Design review of the part built by this model. Coordinates are the model's own, in mm. Face numbers are marked on the shaded views. A direction names the side the tool comes from. Round coordinates to 2 decimals unless told otherwise and drop trailing zeros. Loops run counter-clockwise (first coordinate to the right, second up) from the corner with the lowest first, then second, coordinate; pieces in that order, holes last. Notation, with made-up numbers: M 38,-17 L 96,-17 A8 cw 96,-12 Z; hole C 10,75 d3. An arc over 180 degrees is marked long. Answer as CSV lines item,"result". Start each with the question number.
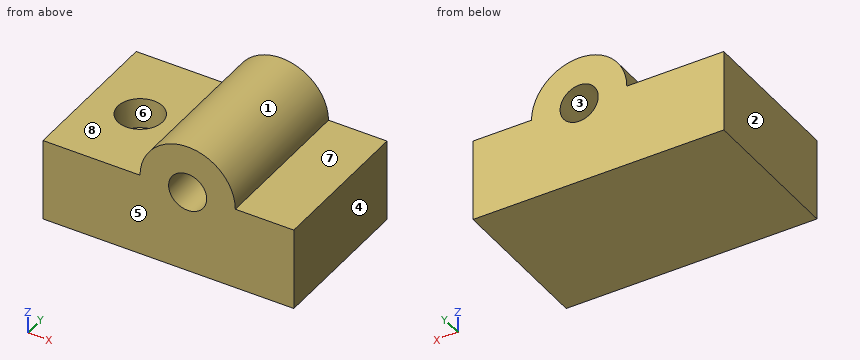
from build123d import *

# Parameters (mm, degrees)
F1_DEPTH = 60
F2_R     = 7.5
F3_DEPTH = 60
F5_R     = 8.827636
F6_DEPTH = 12


with BuildPart() as f1:
    # F0 (on Front) → F1 (new body)
    with BuildSketch(Plane.XZ):
        with BuildLine():
            Line((-98.720774, 0), (0, 0))
            Line((0, 0), (0, 32.434803))
            Line((0, 32.434803), (-22.520235, 32.434803))
            Line((-22.520235, 32.434803), (-23.024651, 32.434803))
            ThreePointArc((-23.024651, 32.434803), (-41.782826, 51.192978), (-60.541002, 32.434803))
            Line((-60.541002, 32.434803), (-61.611962, 32.434803))
            Line((-61.611962, 32.434803), (-98.720774, 32.434803))
            Line((-98.720774, 32.434803), (-98.720774, 0))
        make_face()
    extrude(amount=F1_DEPTH)

    # F2 (on face) → F3 (cut, through all)
    with BuildSketch(Plane.XZ.offset(60)):
        with Locations((-41.782826, 32.434803)):
            Circle(F2_R)
    extrude(amount=-F3_DEPTH, mode=Mode.SUBTRACT)

    # F5 (on face) → F6 (cut)
    with BuildSketch(Plane.XY.offset(32.434803)):
        with Locations((-78.823261, -29.944986)):
            Circle(F5_R)
    extrude(amount=-F6_DEPTH, mode=Mode.SUBTRACT)


solid = f1.part
Item 1: Consider section B-B, the plane y = -20. Write out the cut boundary in (x, z), then the cut area to 3 significant figures.
Item 2: Consider section D-D, the plane z = 47. Write out the cut boundary in (x, y), then the cut area to 3 significant figures.
Item 3: To check wall thickness, follow line 1 (X direction, y = -25.5, z = 28.5); line 2 (X direction, y = -17, z = 33); line 3 (Z direction, x = -8, y = -11.5). State the ranges of each line that lie inside material, in increasing order.
Item 4: Tool access review of the marked faces 4, 5, 6, 7 and 8: name each direction out of +Z, -Z, +X, -X, +Y, -Y from which nothing blocks a thin tool from reaching the whole face with its end or side.
Item 5: Consider section C-C, the plane x = -12. Write out the cut boundary in (y, z), then the cut area to 3 significant figures.
Item 6: Consider section A-A, the plane z = 29. Write out the cut boundary in (x, y), then the cut area to 3 significant figures.
Item 7: The part is to be moulded in two halves that separate along X. For the marked faces 1, 2 and 3, say which applies: +X half, -X half, draft (parallel to the pull), parting line (faces both ways), or undercut.
Item 8: Insertion check: pin 1 Ø4 at (y, z) = (-9, 41.5) entering from -X; pin 2 Ø20.5 at (x, y) = (-78.82, -29.94) entering from +Z. Each pin has a flat end and moves straight along its axis. Give the tip position at first contact, or say it passes through.
Found:
1,outline,"M -98.72,0 L 0,0 L 0,32.43 L -23.02,32.43 A18.76 ccw -60.54,32.43 L -98.72,32.43 Z; hole C -41.78,32.43 d15"
1,area,"3,580 mm^2"
2,outline,"M -53.6,-60 L -29.96,-60 L -29.96,0 L -53.6,0 Z"
2,area,"1,420 mm^2"
3,line 1,"x = -98.72 to -86.45, -71.2 to -48.17, -35.4 to 0"
3,line 2,"x = -60.53 to -49.26, -34.3 to -23.03"
3,line 3,"z = 0 to 32.43"
4,face 4,"+Z, -Z, +X, +Y, -Y"
4,face 5,"+Z, -Z, +X, -X, -Y"
4,face 6,"+Z"
4,face 7,"+Z, +X, +Y, -Y"
4,face 8,"+Z, -X, +Y, -Y"
5,outline,"M -60,0 L 0,0 L 0,32.43 L -60,32.43 Z"
5,area,"1,950 mm^2"
6,outline,"M -98.72,-60 L -48.45,-60 L -48.45,0 L -98.72,0 Z; M -35.12,-60 L 0,-60 L 0,0 L -35.12,0 Z; hole C -78.82,-29.94 d17.66"
6,area,"4,880 mm^2"
7,face 1,"parting line"
7,face 2,"-X half"
7,face 3,"undercut"
8,pin 1,"stops at x = -59.16"
8,pin 2,"stops at z = 32.43"
